Can you work these out from the drawing? Everything is in mm from the part's minimum corner. A direction names the side the tool comes from. Round coordinates to 2 decimals unless told otherwise and drop trailing zeros. Loops run counter-clockwise (first coordinate to the right, second up) from the corner with the lowest first, then second, coordinate; pieces in that order, holes last. Notation, with made-up numbers: M 39,-23.75 L 47,-23.75 A13 cw 47,-2.75 Z; hole C -19,-20 d10. An arc over 180 degrees is marked long. One line per question, with ' | ' between items. Start each with the question number.
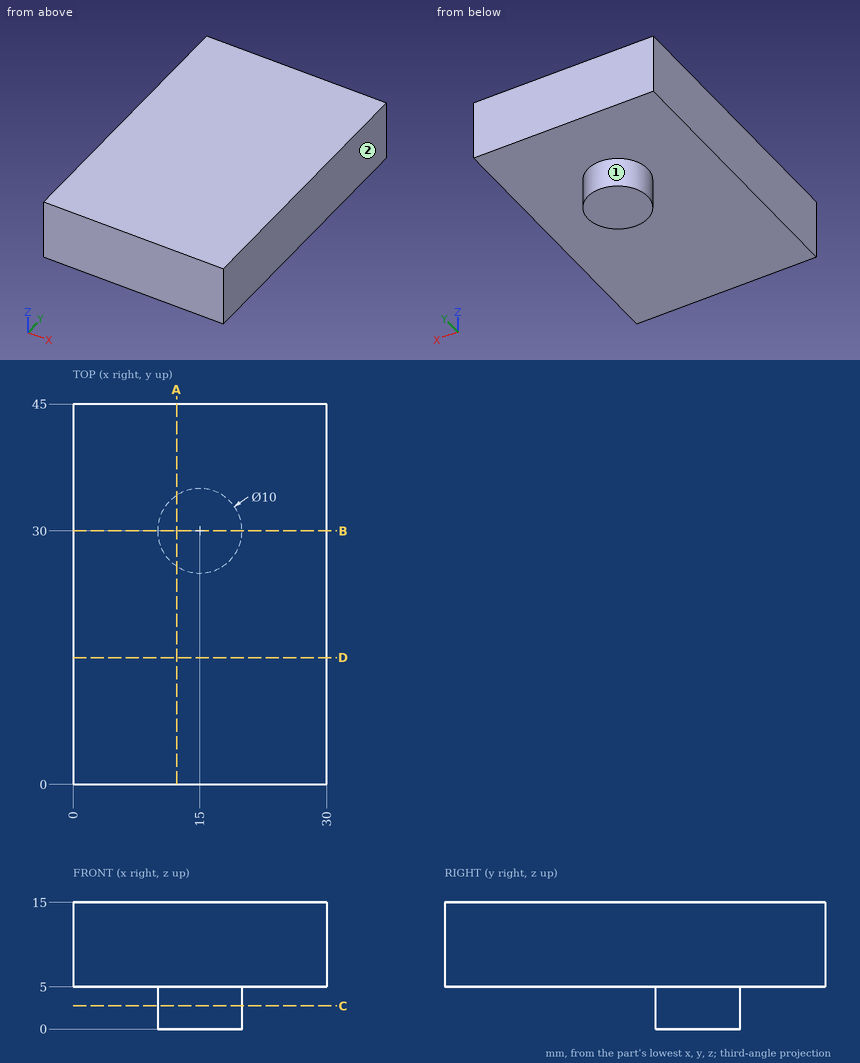
1) Imagine slicing it at C-C (z = 2.75). Write out the boundary of the cut face in (x, y).
2) Please list where these lines run through material, in increasing order: L1, parallel to Z at x = 10.75, y = 34.5; L2, parallel to X at y = 30, z = 1; L3, parallel to X at y = 28, z = 4.5. Write a range as from..to.
3) I'm going to push flat-ended pins straight in: pin 1 Ø8 at (x, z) = (7.5, 8.5) entering from -Y; pin 2 Ø1.5 at (x, y) = (3.5, 18.5) entering from -Z. Where does each tip first touch, or does it pass through?
4) Imagine slicing it at D-D (y = 15). Write out the boundary of the cut face in (x, z), then the cut area to 3 significant figures.
5) Imagine slicing it at A-A (x = 12.25). Write out the boundary of the cut face in (y, z), then the cut area to 3 significant figures.
6) For the marked faces 1 and 2, which set-ups out of +Z, -Z, +X, -X, +Y, -Y let a thin tool reach every point of the face, with its end or its side?
7) Imagine slicing it at B-B (y = 30). Write out the boundary of the cut face in (x, z).
Results are:
1) outline: C 15,30 d10
2) L1: 5..15 | L2: 10..20 | L3: 10.42..19.58
3) pin 1: y = 0 | pin 2: z = 5
4) outline: M 0,5 L 30,5 L 30,15 L 0,15 Z | area: 300 mm²
5) outline: M 0,5 L 25.82,5 L 25.82,0 L 34.18,0 L 34.18,5 L 45,5 L 45,15 L 0,15 Z | area: 492 mm²
6) face 1: -Z | face 2: +Z, -Z, +X, +Y, -Y
7) outline: M 0,5 L 10,5 L 10,0 L 20,0 L 20,5 L 30,5 L 30,15 L 0,15 Z
